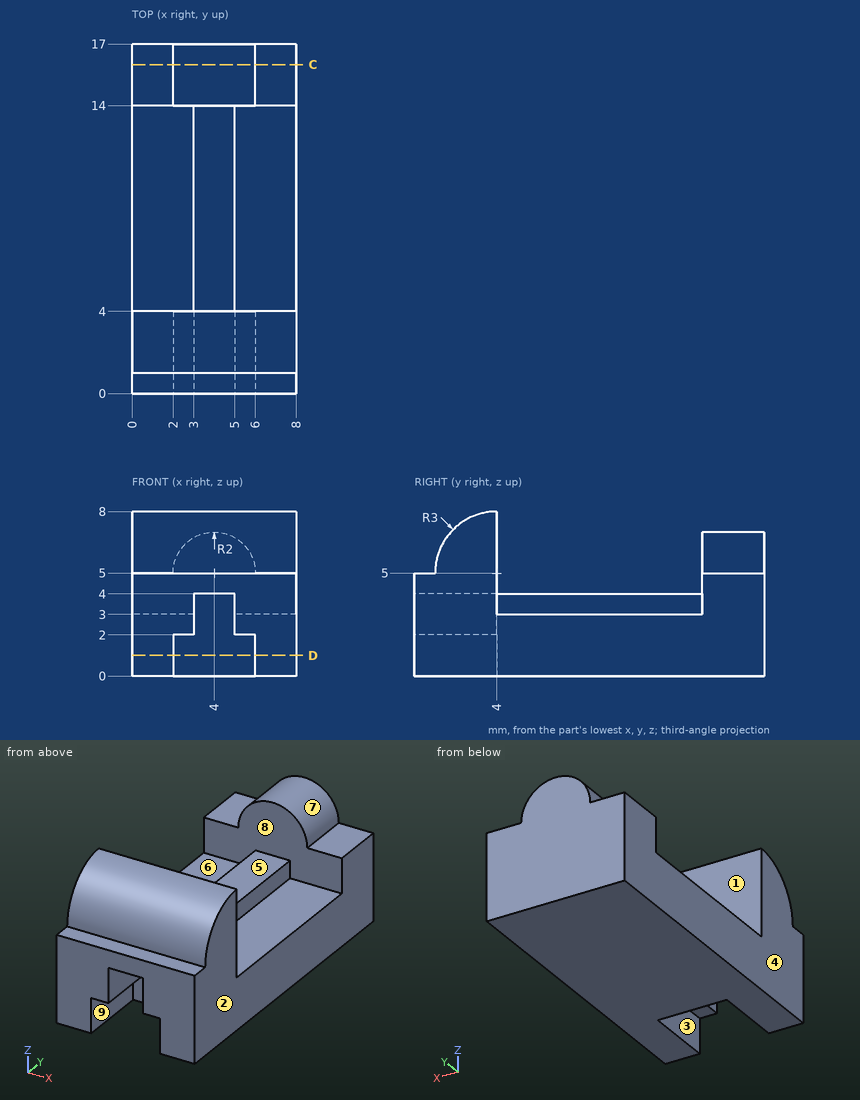
Input: dimensioned drawing with shaded views. Units: mm. Origin: part minimum x, y, z. A direction names the side the tool comes from. Give positions to 0.01 mm unless a question says otherwise; leave off trailing zeros. Write each loop counter-clockwise with the first axis right and the second up, starting at its lowest first coordinate (ties: lowest second). Pieces come first, ordered by that corner, then holes. Notation, with made-up numbers: (-18.5, -10.75) -> (18.5, -10.75) arc R16 cw to (18.5, 15.25) -> close; hole circle Ø10 at (2, 31.5). An arc over 180 degrees is marked (long way). Return JSON: item names as keys, results as strings. Group by question number.
1. Access query for the marked faces 5, 6, 7, 8 and 9. Directions: +Z, -Z, +X, -X, +Y, -Y. A direction counts if a zero-diameter tool reaches every point of the face in a straight line with its end or side. Return the directions, or none.
2. Section C-C, the plane y = 16. Output: boundary loops of the cut face in (x, z), then the cut area to 3 significant figures.
3. Pin query (flat end, axial travel): pin 1 Ø0.8 at (y, z) = (11, 3.5) entering from -X; pin 2 Ø2.5 at (x, y) = (6.5, 11) entering from +Z; pin 3 Ø0.6 at (x, y) = (1, 16) entering from +Z. Return the tip coordinate at first contact, or that it passes through.
4. Material intervals for line 1 (Y direction, x = 1.5, z = 4); line 2 (X direction, y = 1.5, z = 1.25); line 3 (Z direction, x = 2.75, y = 13.75), sorted ascending. Write a range as from..to.
5. Section D-D, the plane z = 1. Output: boundary loops of the cut face in (x, y).
6. Mould query, pull axis X, two halves, no side actions, for the marked faces 1, 2, 3 and 4. Classes: +X half, -X half, draft (parallel to the pull), parting line (faces both ways), or undercut.
Determined:
{
 "1": {"face 5": "+Z, +X, -X", "face 6": "+Z, -X", "face 7": "+Z, +Y", "face 8": "+Z", "face 9": "-Z, -Y"},
 "2": {"outline": "(0, 0) -> (8, 0) -> (8, 5) -> (6, 5) arc R2 ccw to (2, 5) -> (0, 5) -> close", "area": "46.3 mm2"},
 "3": {"pin 1": "stops at x = 3", "pin 2": "stops at z = 3", "pin 3": "stops at z = 5"},
 "4": {"line 1": "y = 0..4, 14..17", "line 2": "x = 0..2, 6..8", "line 3": "z = 0..3"},
 "5": {"outline": "(0, 0) -> (2, 0) -> (2, 4) -> (6, 4) -> (6, 0) -> (8, 0) -> (8, 17) -> (0, 17) -> close"},
 "6": {"face 1": "draft", "face 2": "+X half", "face 3": "undercut", "face 4": "-X half"}
}
